Can you work these out from the model? Positions are in its coordinate system, mm. A direction names the side the tool comes from. Coordinates: 2 decimals unless noted, no trailing zeros. Use a Markdown table: item, result. Add a question column.
(1) I want a section at A-A (y = -0.85). State how many separate pieces and enclosed holes the cut face has, and give its area (3 significant figures).
(2) For pin 1 Ø1.5 at (y, z) = (-1, 1.5) entering from -X; pin 2 Ø1.5 at (x, y) = (-5, -2) entering from +Z; pin 3 Ø1 at (x, y) = (-11.5, -2) entering from -Z; pin 4 Ø4 at (x, z) = (-12.9, -8.91) entering from -Y, each with a flat end and sliding along its axis, tell me the tip position at first contact or that it passes through.
(3) We'd pull the mould along X, two halves only. Please class faces 4 (the flat face through (0, 0, -20)), 5 (the flat face through (-15.4, -1, 1)), 6 (the flat face through (1.5, -1, -9)): pulls with the +X half, pulls with the -X half, needs draft (parallel to the pull), parting line crosses it, or undercut.
(4) On a 3-axis mill with a long thin cutter (end or side, diameter ignored), from which of +Z, -Z, +X, -X, +Y, -Y can I reach the whole of each face in a straight line? I mean faces 1 (the flat face through (15.4, -1, 1)), 2 (the flat face through (-20, -1, 0)), 3 (the flat face through (11.59, -1, 1)). Say none if no direction works.
(5) If I drill on L1, parallel to X at y = -2.9, z = -0.5; L2, parallel to X at y = -0.55, z = 1; L3, parallel to Z at x = 12.9, y = -1.7, over which ranges is the centre line in solid material (lowest first)? Write a range as [from, to].
```python
from build123d import *

# Parameters (mm, degrees)
F0_R     = 1.5
F0_W     = 3.81
F0_H     = 3
F1_DEPTH = 3


# Not quite as in the source:
# - a feature names something its author has since deleted; it is built from what else it names


with BuildPart() as f1:
    # F0 (on Front) → F1 (new body)
    with BuildSketch(Plane.XZ):
        with BuildLine():
            Line((-1.5, -18.6309), (-1.5, 0))
            Line((-1.5, 0), (-7.59, 0))
            Line((-7.59, 0), (-11.59, 0))
            Line((-11.59, 0), (-15.4, 0))
            Line((-15.4, 0), (-17.05, 0))
            Line((-17.05, 0), (-25.4, 0))
            add(Edge.make_bspline(
                [(-25.4, 0), (-25.4, -30), (-12.7, -37.25), (0, -37.25)],
                knots=[0, 0, 0, 0, 0.5, 0.5, 0.5, 0.5], degree=3))
            Line((0, -37.25), (0, -18.6309))
            Line((0, -18.6309), (-1.5, -18.6309))
        make_face()
        with Locations((-12.9, -8.9107090607)):
            Circle(F0_R, mode=Mode.SUBTRACT)
        with BuildLine():
            Line((4.35, 0), (1.5, 0))
            Line((1.5, 0), (1.5, -18.6309))
            Line((1.5, -18.6309), (0, -18.6309))
            Line((0, -18.6309), (0, -37.25))
            add(Edge.make_bspline(
                [(0, -37.25), (12.7, -37.25), (25.4, -30), (25.4, 0)],
                knots=[0.5, 0.5, 0.5, 0.5, 1, 1, 1, 1], degree=3))
            Line((25.4, 0), (15.4, 0))
            Line((15.4, 0), (11.59, 0))
            Line((11.59, 0), (6.35, 0))
            Line((6.35, 0), (4.35, 0))
        make_face()
        with Locations((12.9, -8.9107090607)):
            Circle(F0_R, mode=Mode.SUBTRACT)
        with Locations((13.495, 1.5)):
            Rectangle(F0_W, F0_H)
        with Locations((-13.495, 1.5)):
            Rectangle(F0_W, F0_H)
    extrude(amount=F1_DEPTH)


solid = f1.part
```
Answers follow:
| question | item | result |
|---|---|---|
| 1 | separate pieces | 1 |
| 1 | enclosed holes | 2 |
| 1 | area | 1,530 mm² |
| 2 | pin 1 | stops at x = -15.4 |
| 2 | pin 2 | stops at z = 0 |
| 2 | pin 3 | stops at z = -34.92 |
| 2 | pin 4 | stops at y = -3 |
| 3 | face 4 | needs draft |
| 3 | face 5 | pulls with the -X half |
| 3 | face 6 | undercut |
| 4 | face 1 | +Z, +X, +Y, -Y |
| 4 | face 2 | +Z, -X, +Y, -Y |
| 4 | face 3 | +Z, +Y, -Y |
| 5 | L1 | x = [-25.4, -1.5], [1.5, 25.4] |
| 5 | L2 | x = [-15.4, -11.59], [11.59, 15.4] |
| 5 | L3 | z = [-33.85, -10.41], [-7.41, 3] |
